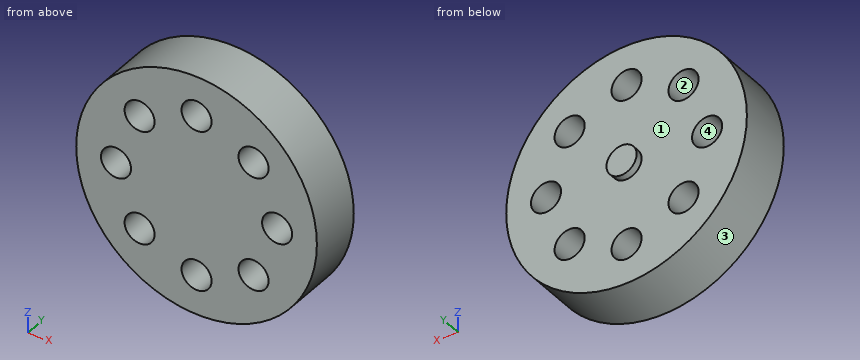
```python
from build123d import *

# Parameters (mm, degrees)
F0_R     = 12.7
F0_R_2   = 1.5875
F0_R_3   = 6.35
F0_R_4   = 3.175
F1_DEPTH = 5.588
F2_R     = 1.5875
F3_DEPTH = 6.35


with BuildPart() as f1:
    # F0 (on Front) → F1 (new body)
    with BuildSketch(Plane.XZ):
        Circle(F0_R)
        with Locations((-6.0124402351, -6.0124402351)):
            Circle(F0_R_2, mode=Mode.SUBTRACT)
        with Locations((0, -8.5028745234)):
            Circle(F0_R_2, mode=Mode.SUBTRACT)
        with Locations((6.0124402351, -6.0124402351)):
            Circle(F0_R_2, mode=Mode.SUBTRACT)
        with Locations((-8.5028745234, 0)):
            Circle(F0_R_2, mode=Mode.SUBTRACT)
        with Locations((-6.0124402351, 6.0124402351)):
            Circle(F0_R_2, mode=Mode.SUBTRACT)
        Circle(F0_R_3, mode=Mode.SUBTRACT)
        with Locations((6.0124402351, 6.0124402351)):
            Circle(F0_R_2, mode=Mode.SUBTRACT)
        with Locations((8.5028745234, 0)):
            Circle(F0_R_2, mode=Mode.SUBTRACT)
        with Locations((0, 8.5028745234)):
            Circle(F0_R_2, mode=Mode.SUBTRACT)
        Circle(F0_R_3)
        Circle(F0_R_4, mode=Mode.SUBTRACT)
        Circle(F0_R_4)
    extrude(amount=-F1_DEPTH)

    # F2 (on Front) → F3 (join)
    with BuildSketch(Plane.XZ):
        Circle(F2_R)
    extrude(amount=-F3_DEPTH)


solid = f1.part
```
The listing builds one solid part. Answer for the finished solid, in the listing's coordinates (mm). Face numbers are marked on the shaded views. Round coordinates to 2 decimals unless told otherwise and drop trailing zeros. Loops run counter-clockwise (first coordinate to the right, second up) from the corner with the lowest first, then second, coordinate; pieces in that order, holes last.
Q1. Section B-B, the plane x = 0 is taken. Determine the outline of the cut face in (y, z).
Q2. Section D-D, the plane x = -8 is taken. Determine the outline of the cut face in (y, z).
Q3. Section C-C, the plane y = 4.5 is taken. Count the separate pieces of the cut face and the enclosed holes in it, then the cut area to 3 significant figures.
Q4. For a pull along Z with two mould halves and no side action, classify the marked faces 1, 2, 3 and 4 as released by +Z, released by -Z, zero draft, split by the parting line, or undercut.
Q5. Section A-A, the plane z = 0 is taken. Determine the outline of the cut face in (x, y).
Q6. Find the intervals of material crossed by line 1 (Z direction, x = 6, y = 0.5); line 2 (X direction, y = 1, z = -0.5); line 3 (X direction, y = 4.5, z = -5.5), in increasing order.
Q7. Given pin 1 Ø1.9 at (x, z) = (-6.01, 6.01) entering from -Y; pin 2 Ø1.5 at (x, z) = (5, 1.5) entering from +Y; pin 3 Ø2 at (y, z) = (1, 10) entering from -X; pin 4 Ø1 at (y, z) = (1, 4) entering from +X, each flat-ended and moving along its own axis, determine where each tip first touches the part or whether it passes through.
Completed:
1. outline: (0, -12.7) - (5.59, -12.7) - (5.59, -10.09) - (0, -10.09) - close; (0, -6.92) - (5.59, -6.92) - (5.59, -1.59) - (6.35, -1.59) - (6.35, 1.59) - (5.59, 1.59) - (5.59, 6.92) - (0, 6.92) - close; (0, 10.09) - (5.59, 10.09) - (5.59, 12.7) - (0, 12.7) - close
2. outline: (0, -9.86) - (5.59, -9.86) - (5.59, -1.51) - (0, -1.51) - close; (0, 1.51) - (5.59, 1.51) - (5.59, 9.86) - (0, 9.86) - close
3. separate pieces: 1
3. enclosed holes: 8
3. area: 443 mm2
4. face 1: zero draft
4. face 2: undercut
4. face 3: split by the parting line
4. face 4: undercut
5. outline: (-12.7, 0) - (-10.09, 0) - (-10.09, 5.59) - (-12.7, 5.59) - close; (-6.92, 0) - (6.92, 0) - (6.92, 5.59) - (1.59, 5.59) - (1.59, 6.35) - (-1.59, 6.35) - (-1.59, 5.59) - (-6.92, 5.59) - close; (10.09, 0) - (12.7, 0) - (12.7, 5.59) - (10.09, 5.59) - close
6. line 1: z = -11.19 to -7.6, -4.42 to 4.42, 7.6 to 11.19
6. line 2: x = -12.69 to -10.01, -7 to 7, 10.01 to 12.69
6. line 3: x = -11.45 to -7.51, -4.51 to 4.51, 7.51 to 11.45
7. pin 1: passes through
7. pin 2: stops at y = 5.59
7. pin 3: stops at x = -8.96
7. pin 4: stops at x = 12.21
